Here's the drawing with two shaded views (mm, measured from the low corner). I have some questions. Give positions to 0.01 mm unless a question says otherwise; leave off trailing zeros. Write each loop counter-clockwise with the first axis right and the second up, starting at its lowest first coordinate (ties: lowest second). Pieces come first, ordered by that corner, then holes. Notation, with made-up numbers: (-25.5, 68) - (-20.5, 68) arc R19 cw to (-20.5, 79) - close; hole circle Ø11 at (54, 5). An arc over 180 degrees is marked (long way). Write item = value, one per line.
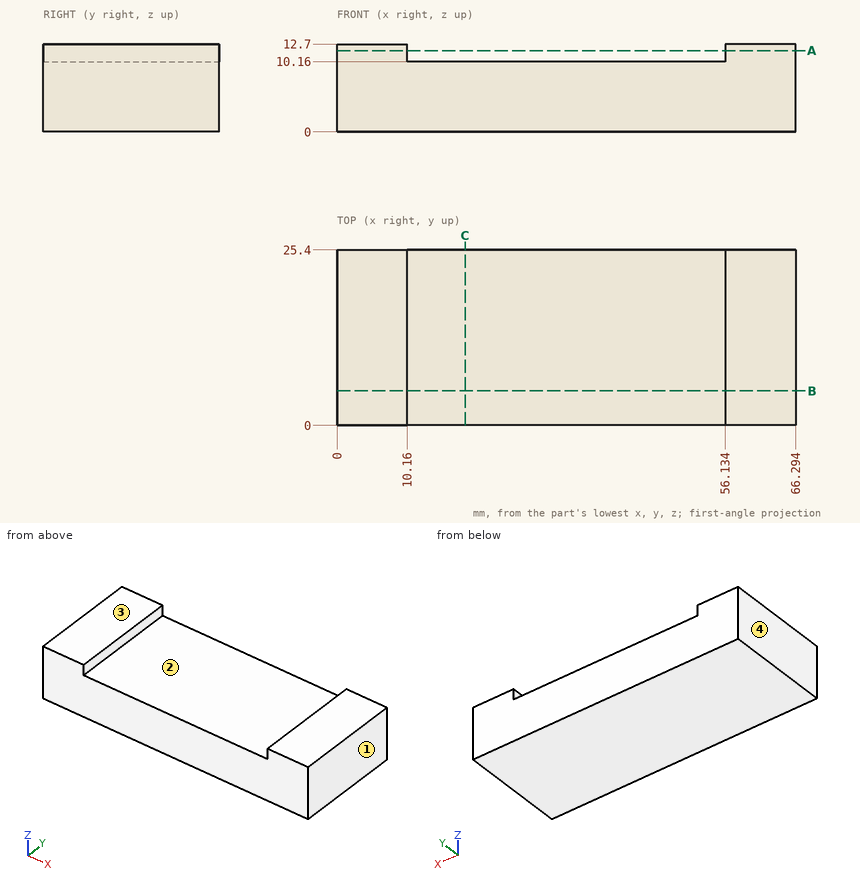
1. I need wall thicknesses on line 1 (X direction, y = 18.25, z = 12.25); line 2 (Z direction, x = 21.5, y = 1.5). Which ranges of each line are inside material? Lowest first, please.
Filled sheet:
line_1 = 0 to 10.16, 56.13 to 66.29
line_2 = 0 to 10.16
2. If we section it at C-C, the plane x = 18.5: Please give me the cut outline in (y, z), and give its area (3 significant figures).
Filled sheet:
outline = (0, 0) - (25.4, 0) - (25.4, 10.16) - (0, 10.16) - close
area = 258 mm2
3. For pin 1 (12.5 mm diameter, centred on x = 44, y = 7.5, fed in from +Z), with a flat end and sliding along its axis, tell me the tip position at first contact or that it passes through.
Filled sheet:
pin_1 = 10.16
4. If we section it at A-A, the plane z = 11.75: Please give me the cut outline in (x, y), and give its area (3 significant figures).
Filled sheet:
outline = (0, 0) - (10.16, 0) - (10.16, 25.4) - (0, 25.4) - close; (56.13, 0) - (66.29, 0) - (66.29, 25.4) - (56.13, 25.4) - close
area = 516 mm2
5. Thinking about a two-plate mould opening in X: for the marked faces 1, 2, 3 and 4, which applies, pulls with the +X half, pulls with the -X half, needs draft (parallel to the pull), parting line crosses it, or undercut?
Filled sheet:
face_1 = pulls with the +X half
face_2 = undercut
face_3 = needs draft
face_4 = pulls with the -X half
6. If we section it at B-B, the plane y = 5: Please give me the cut outline in (x, z).
Filled sheet:
outline = (0, 0) - (66.29, 0) - (66.29, 12.7) - (56.13, 12.7) - (56.13, 10.16) - (10.16, 10.16) - (10.16, 12.7) - (0, 12.7) - close
